Geometry: final body of the model. Coordinates: model frame, mm. Give positions to 0.01 mm unless a question says otherwise; leave off trailing zeros. Loops run counter-clockwise (first coordinate to the right, second up) from the corner with the lowest first, then second, coordinate; pieces in that order, holes last. Notation, with made-up numbers: (-13.75, -14.75) - (-9.75, -14.75) arc R17 cw to (-9.75, -8.75) - close; hole circle Ø3 at (-21.5, 81.5). An arc over 180 degrees is marked (long way). Use one line per item in the form item = value.
```python
from build123d import *

# Parameters (mm, degrees)
SKETCH3_R           = 68.58
SKETCH3_R_2         = 65.405
BOSS_EXTRUDE1_DEPTH = 3.175
SKETCH4_R           = 0.79375
CUT_EXTRUDE1_DEPTH  = 98.038721266
CIRPATTERN1_COUNT   = 4


with BuildPart() as part:
    # Sketch3 → Boss-Extrude1 (new, symmetric)
    with BuildSketch(Plane.XY):
        Circle(SKETCH3_R)
        Circle(SKETCH3_R_2, mode=Mode.SUBTRACT)
    extrude(amount=BOSS_EXTRUDE1_DEPTH, both=True)

    # Sketch4 → Cut-Extrude1 (cut, through all)
    with BuildSketch(Plane(origin=(0, 0, 0), x_dir=(1, 0, 0), z_dir=(0, 1, 0))):
        with Locations(Location((0, 0, 0), (0, 0, 270))):
            Circle(SKETCH4_R)
    cut_extrude1 = extrude(amount=-CUT_EXTRUDE1_DEPTH, mode=Mode.SUBTRACT)

    # CirPattern1: Cut-Extrude1 ×4 about axis
    cirpattern1_axis = Axis((0, 0, 3.175), (0, 0, -1))
    for i in range(1, CIRPATTERN1_COUNT):
        add(cut_extrude1.rotate(cirpattern1_axis, i * 360 / CIRPATTERN1_COUNT), mode=Mode.SUBTRACT)


solid = part.part
```
(1) Pin query (flat end, axial travel): P1, Ø1.4, axis at y = 0, z = 0, coming from the -X side; P2, Ø1, axis at y = 30, z = 2.5, coming from the +X side; P3, Ø1.5, axis at x = -36.5, z = -2.5, coming from the -Y side. Return the tip coordinate at first contact, or that it passes through.
Solution:
P1 = through
P2 = 61.91
P3 = -58.52
(2) Cut plane A-A (y = 29). Return the cut outline in (x, z) (3 decimals).
Solution:
outline = (-62.147, -3.175) - (-58.624, -3.175) - (-58.624, 3.175) - (-62.147, 3.175) - close; (58.624, -3.175) - (62.147, -3.175) - (62.147, 3.175) - (58.624, 3.175) - close
(3) Material intervals for L1, parallel to X at y = 0, z = 1 (3 decimals); L2, parallel to Z at x = 0, y = -67.3 (3 decimals); L3, parallel to Y at x = -43, z = 2.25, sorted ascending. Write a range as from..to.
Solution:
L1 = -68.58..-65.405, 65.405..68.58
L2 = -3.175..-0.794, 0.794..3.175
L3 = -53.42..-49.28, 49.28..53.42
(4) Cut plane B-B (x = 52). Return the cut outline in (y, z) (3 decimals), plus the area to 3 significant figures.
Solution:
outline = (-44.713, -3.175) - (-39.671, -3.175) - (-39.671, 3.175) - (-44.713, 3.175) - close; (39.671, -3.175) - (44.713, -3.175) - (44.713, 3.175) - (39.671, 3.175) - close
area = 64.0 mm2
(5) Cut plane C-C (z = 1.75). Return the cut outline in (x, y) (3 decimals), plus the area to 3 significant figures.
Solution:
outline = circle Ø137.16 at (0, 0); hole circle Ø130.81 at (0, 0)
area = 1,340 mm2
(6) Pull-direction query (Y, two-part tool) for faces 1 (the face through (61, -25, 3.175)), 2 (the face through (-14.18, -63.85, -0.04)), 3 (the face through (36.868, 57.827, 0.044)); classes: released by +Y, released by -Y, zero draft, split by the parting line, or undercut.
Solution:
face_1 = zero draft
face_2 = undercut
face_3 = split by the parting line
